Autodesk Inventor part; units mm, degrees
ref_plane "YZ Plane" through (0, 0, 0) normal (1, 0, 0) x (0, 1, 0)
ref_plane "XZ Plane" through (0, 0, 0) normal (0, 1, 0) x (-1, 0, 0)
ref_plane "XY Plane" through (0, 0, 0) normal (0, 0, 1) x (1, 0, 0)
sketch "Sketch1" plane through (0, 0, 0) normal (0, 1, 0) x (-1, 0, 0)
  circle A0 centre (0, 0) radius 14.351 construction
  line L0 (-12.7, -34.925) -> (12.7, -34.925) construction
  circle A1 centre (0, 0) radius 22.225 construction
  circle A2 centre (0, 0) radius 31.75 construction
  circle A3 centre (-15.875, -27.4963) radius 4.7625 construction
  arc A4 (-20.4289, -28.8903) -> (-25.4478, -18.9862) centre (-51.4511, -38.3868) ccw construction
  arc A5 (-3.7186, -31.5315) -> (-14.8053, -32.1371) centre (-7.5184, -63.7513) ccw construction
  line L1 (0, 0) -> (0, -22.225) construction
  circle A6 centre (15.875, -27.4963) radius 4.7625 construction
  arc A7 (25.4478, -18.9862) -> (20.4289, -28.8903) centre (51.4511, -38.3868) ccw construction
  arc A8 (14.8053, -32.1371) -> (3.7186, -31.5315) centre (7.5184, -63.7513) ccw construction
  circle A9 centre (-12.7, -34.925) radius 2.5527 construction
  circle A10 centre (-12.7, -34.925) radius 3.1548 construction
  circle A11 centre (12.7, -34.925) radius 3.1548 construction
  line L2 (-16, -53.9) -> (16, -53.9) construction
  circle A12 centre (0, 0) radius 53.9 construction
  circle A13 centre (0, -40.64) radius 2.5527 construction
  circle A14 centre (12.7, -41.91) radius 2.5527 construction
  point P0 (0, -34.925)
  point P1 (31.75, 0)
  point P2 (15.875, 27.4963)
  point P3 (-15.875, 27.4963)
  point P4 (-31.75, 0)
  point P5 (15.875, -27.4963)
  point P6 (0, -53.9)
  point P7 (0, -53.9)
  point P8 (-12.7, -41.91)
  dimension "d3" = 44.45
  dimension "d16" = 107.8
  dimension "d0" = 28.702
  dimension "d1" = 25.4
  dimension "d2" = 34.925
  dimension "d4" = 63.5
  dimension "d7" = 360
  dimension "d9" = 9.525
  dimension "d10" = 32.4431
  dimension "d11" = 32.4431
  dimension "d12" = 5.1054
  dimension "d14" = 0.6021
  dimension "d15" = 32
  dimension "d18" = 40.64
  dimension "d19" = 5.1054
  dimension "d20" = 6.985
  dimension "d21" = 5.1054
sketch "Sketch2" plane through (0, 0, 0) normal (0, 1, 0) x (-1, 0, 0)
  circle A0 centre (12.7, -41.91) radius 2.5527 construction
  circle A1 centre (12.7, -41.91) radius 5.7277 construction
  circle A2 centre (16, -53.9) radius 5.7277 construction
  line L0 (18.2224, -40.3901) -> (21.5224, -52.3801)
  circle A3 centre (-12.7, -41.91) radius 5.7277 construction
  circle A4 centre (-16, -53.9) radius 5.7277 construction
  line L1 (12.7, -36.1823) -> (-12.7, -36.1823)
  line L2 (-18.2224, -40.3901) -> (-21.5224, -52.3801)
  line L3 (-16, -59.6277) -> (16, -59.6277)
  arc A5 (18.2224, -40.3901) -> (12.7, -36.1823) centre (12.7, -41.91) ccw
  arc A6 (16, -59.6277) -> (21.5224, -52.3801) centre (16, -53.9) ccw
  arc A7 (-21.5224, -52.3801) -> (-16, -59.6277) centre (-16, -53.9) ccw
  arc A8 (-12.7, -36.1823) -> (-18.2224, -40.3901) centre (-12.7, -41.91) ccw
  line L4 (-12, -59.6277) -> (-12, -44.1197) construction
  line L5 (-12, -44.1197) -> (12, -44.1197) construction
  line L6 (12, -44.1197) -> (12, -59.6277) construction
  line L7 (12, -59.6277) -> (-12, -59.6277)
  line L8 (11, -44.1197) -> (-11, -44.1197)
  line L9 (-11, -44.1197) -> (-12, -59.6277)
  line L10 (11, -44.1197) -> (12, -59.6277)
  point P0 (0, 0)
  point P1 (0, -59.6277)
  point P2 (12, -59.6277)
  point P3 (0, -44.1197)
  point P4 (0, -44.1197)
  point P5 (12, -59.6277)
  dimension "d22" = 5.1054
  dimension "d23" = 3.175
  dimension "d40" = 24
  dimension "d41" = 15.508
  dimension "d45" = 22
extrude "Extrusion1" add sketch "Sketch2" against normal blind 9.525
hole "Hole1" at (-12.7, 0, -41.91) at (12.7, 0, -41.91) direction (0, -1, 0) diameter 5.1054 end through all
hole "Hole2" at (16, 0, -53.9) at (-16, 0, -53.9) direction (0, -1, 0) diameter 2.6416 end through all
sketch "Sketch3" plane through (0, -9.525, 0) normal (0, -1, 0) x (1, 0, 0)
  point P0 (0, 0)
sketch "Sketch4" plane through (16, 0, -59.6277) normal (0, 0, -1) x (-1, 0, 0)
  line L0 (28.7, 0) -> (3.3, 0) construction
  line L1 (5, 0) -> (27, 0)
  line L2 (27, 0) -> (28, -9.525)
  line L3 (28, -9.525) -> (4, -9.525)
  line L4 (3.3, -9.525) -> (28.7, -9.525) construction
  line L5 (4, -9.525) -> (5, 0)
  point P0 (16, 0)
  point P1 (16, 0)
  point P2 (16, -9.525)
  point P3 (16, -9.525)
  dimension "d46" = 22
  dimension "d47" = 24
extrude "Extrusion3" cut sketch "Sketch4" against normal blind 14
fillet "Fillet2" radius 3.175 4 edges at (11.5, -4.7625, -45.6277) (-11.5, -4.7625, -45.6277) (-11.5, -4.7625, -59.6277) (11.5, -4.7625, -59.6277)
sketch "Sketch5" plane through (0, 0, 0) normal (1, 0, 0) x (0, 1, 0)
  line L0 (-9.525, -45.6277) -> (-9.525, -36.1823) construction
  line L1 (-9.525, -36.1823) -> (0, -36.1823) construction
  line L2 (0, -36.1823) -> (0, -45.6277) construction
  line L3 (0, -45.6277) -> (-9.525, -45.6277) construction
  line L4 (0, -59.6277) -> (-6, -59.6277)
  line L5 (-6, -59.6277) -> (-6, -46.6277)
  line L6 (-6, -46.6277) -> (0, -46.6277)
  line L7 (0, -46.6277) -> (0, -59.6277)
  line L8 (-9.525, -59.6277) -> (0, -59.6277) construction
  line L9 (-9.525, -56.4527) -> (-9.525, -48.8027) construction
  point P0 (0, 0)
  dimension "d55" = 6
  dimension "d56" = 13
extrude "Extrusion4" cut sketch "Sketch5" along normal blind 25.4
equation "\"d11\" = d10"
properties part number "AR-020" material "ABS Plastic"
Input: part model. Units: mm. Frame: model coordinates. A direction names the side the tool comes from. Coordinates: 2 decimals unless noted, no trailing zeros. Loops run counter-clockwise (first coordinate to the right, second up) from the corner with the lowest first, then second, coordinate; pieces in that order, holes last.
Q1. Cut plane A-A (z = -55.75). Output: boundary loops of the cut face in (x, y) (3 decimals).
Q2. Cut plane C-C (z = -50.75). Output: boundary loops of the cut face in (x, y) (3 decimals), then the cut area to 3 significant figures.
Q3. Draft query along Z for faces 1 (the face through (20.6, -7.74, -57.31)), 2 (the face through (-19.85, -4.7, -46.3)), 3 (the face through (14.3, -4.8, -43.9)), 4 (the face through (-12.47, -4.9, -58.72)). Return one class per face: +Z half, -Z half, draft (parallel to the pull), parting line (faces both ways), or undercut.
Q4. Cut plane B-B (x = -6.5). Output: boundary loops of the cut face in (y, z) (3 decimals).
Q5. Cut plane D-D (y = -4). Give the number of separate pieces and of enclosed holes in the cut face, then the cut area to 3 significant figures.
Q6. Contact query for flat-ended pins moving along their axis: pin 1 (1 mm diameter, centred on y = -6.5, z = -48, fed in from +X); pin 2 (3 mm diameter, centred on y = -5.5, z = -40.5, fed in from -X); pin 3 (1.5 mm diameter, centred on x = 7, y = -4, fed in from -Z); pin 4 (1.6 mm diameter, centred on x = 16, z = -53.9, fed in from -Y). Output: stop coordinate, or through.
Q7. Material intervals for line 1 (X direction, y = -0.25, z = -43.25); line 2 (X direction, y = -6, z = -41); line 3 (Z direction, x = 12.7, y = -4.75), sorted ascending.
Q8. Set-up query: faces 5 (the face through (15, -3, -46.628)), 6 (the face through (-15.2, -4.83, -54.95)), 7 (the face through (-11.493, -4.696, -52.681)). Return all of +Z, -Z, +X, -X, +Y, -Y with unobstructed straight access to the full face (end or side cutting, diameter ignored); none if empty.
Working result:
1. outline: (-21.421, -9.525) - (-12, -9.525) - (-11, 0) - (-21.421, 0) - close; (11.63, -6) - (12, -9.525) - (21.421, -9.525) - (21.421, -6) - close
2. outline: (-21.074, -9.525) - (-12, -9.525) - (-11, 0) - (-21.074, 0) - close; (11.63, -6) - (12, -9.525) - (21.074, -9.525) - (21.074, -6) - close
2. area: 124 mm2
3. face 1: parting line
3. face 2: +Z half
3. face 3: undercut
3. face 4: -Z half
4. outline: (-9.525, -45.628) - (0, -45.628) - (0, -36.182) - (-9.525, -36.182) - close
5. separate pieces: 1
5. enclosed holes: 3
5. area: 433 mm2
6. pin 1: stops at x = 20.45
6. pin 2: stops at x = -18.67
6. pin 3: stops at z = -45.63
6. pin 4: passes through
7. line 1: x = -19.01 to -14.87, -10.53 to 10.53, 14.87 to 19.01
7. line 2: x = -18.39 to -15.08, -10.32 to 10.32, 15.08 to 18.39
7. line 3: z = -46.63 to -44.46, -39.36 to -36.18
8. face 5: -Z, +X, +Y
8. face 6: +Y, -Y
8. face 7: -Z, -Y
